The model under review builds one solid part; all positions refer to its coordinate system, in mm. Coordinates: 2 decimals unless noted, no trailing zeros. Order: outer loops, then holes, each group sorted by start corner. A loop starts at its lowest first (then second) coordinate and runs counter-clockwise, first axis right, second up. Notation, with made-up numbers: (53, -3.5) -> (72, -3.5) arc R28 ccw to (72, 26.5) -> close; hole circle Ø8 at (18, 35). An arc over 180 degrees is marked (long way). Use one line per item in the form item = value.
from build123d import *

# Parameters (mm, degrees)
SKETCH_1_W          = 216
SKETCH_1_H          = 260
EXTRUDE_1_DEPTH     = 2
SKETCH_2_W          = 100
SKETCH_2_H          = 40
CUT_EXTRUDE_1_DEPTH = 2
MM_2_D              = 5


with BuildPart() as part:
    # 草图1 → 凸台-拉伸1 (new body)
    with BuildSketch(Plane(origin=(0, 0, 0), x_dir=(1, 0, 0), z_dir=(0, 1, 0))):
        Rectangle(SKETCH_1_W, SKETCH_1_H)
    extrude(amount=EXTRUDE_1_DEPTH)

    # 草图2 → 切除-拉伸1 (cut)
    with BuildSketch(Plane.XZ):
        with Locations((-1.889005497, -80)):
            Rectangle(SKETCH_2_W, SKETCH_2_H)
    extrude(amount=-CUT_EXTRUDE_1_DEPTH, mode=Mode.SUBTRACT)

    # 大小mm 暗销孔2 (through all)
    with Locations(Plane(origin=(45.636831669, 0, 442.05931397), x_dir=(-0.0785283775902434, 0, -0.9969118787099711), z_dir=(0, -1, 0))):
        with Locations((559.93638869, 93.623184237), (567.396584561, -1.08344424), (574.856780432, -95.790072718), (313.699154648, 74.226674972), (321.159350519, -20.479953505), (328.61954639, -115.186581983)):
            Hole(MM_2_D / 2)


solid = part.part
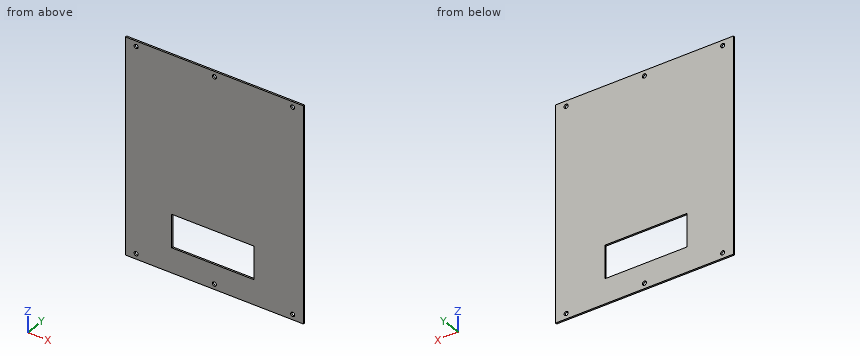
Item 1: To check wall thickness, follow L1, parallel to X at y = 1.4, z = -123.5; L2, parallel to Z at x = 95, y = 1.45; L3, parallel to X at y = 1.1, z = -89.5. State the ranges of each line that lie inside material, in increasing order. Write a range as from..to.
Results found:
L1 = -108..-97.5, -92.5..-2.5, 2.5..92.5, 97.5..108
L2 = -130..-126, -121..121, 126..130
L3 = -108..-51.89, 48.11..108
Item 2: We need section A-A (x = -9). Write out the cut boundary in (y, z), plus the area to 3 significant figures.
Results found:
outline = (0, -130) -> (2, -130) -> (2, -100) -> (0, -100) -> close; (0, -60) -> (2, -60) -> (2, 130) -> (0, 130) -> close
area = 440 mm²
Item 3: We need section B-B (y = 1.05). Write out the cut boundary in (x, z), plus the area to 3 significant figures.
Results found:
outline = (-108, -130) -> (108, -130) -> (108, 130) -> (-108, 130) -> close; hole circle Ø5 at (-95, -123.5); hole circle Ø5 at (-95, 123.5); hole (-51.89, -100) -> (48.11, -100) -> (48.11, -60) -> (-51.89, -60) -> close; hole circle Ø5 at (0, -123.5); hole circle Ø5 at (0, 123.5); hole circle Ø5 at (95, -123.5); hole circle Ø5 at (95, 123.5)
area = 52,000 mm²
Item 4: Clearance check with a flat-ended pin moving along its axis: pin 1 (4 mm diameter, centred on x = -95, z = 123.5, fed in from +Y). State where the tip first meets the part, or that it passes through.
Results found:
pin_1 = through
